```python
from build123d import *

# Parameters (mm, degrees)
F3_R = 0.5
F4_R = 1.25


with BuildPart() as f2:
    # F2: sweep along a path in F1
    with BuildLine(Plane.XY) as f2_path:
        Line((0, 0), (0, 2))
    # F0 (on Front) → F2 (sweep)
    with BuildSketch(Plane.XZ):
        Polygon((-0.5872089498, 2.8263968197), (-2.741335922, 0.904660542), (-2.1541269722, -1.9217362777), (0.5872089498, -2.8263968197), (2.741335922, -0.904660542), (2.1541269722, 1.9217362777), align=None)
    sweep(path=f2_path.line)

    # F3
    f3_edges = [f2.edges().sort_by_distance(p)[0] for p in [
        (-2.447731, 0, -0.508538),
        (-1.664272, 0, 1.865529),
        (0.783459, 0, 2.374067),
        (2.447731, 0, 0.508538),
        (1.664272, 0, -1.865529),
        (-0.783459, 0, -2.374067),
        (-1.664272, 2, 1.865529),
        (0.783459, 2, 2.374067),
        (2.447731, 2, 0.508538),
        (1.664272, 2, -1.865529),
        (-0.783459, 2, -2.374067),
        (-2.447731, 2, -0.508538),
    ]]
    fillet(f3_edges, radius=F3_R)

    # F6: sweep along a path in F5
    with BuildLine(Plane.XY) as f6_path:
        Line((0, -0.6415657117), (0, 2.5134647731))
    # F4 (on Front) → F6 (sweep, cut)
    with BuildSketch(Plane.XZ):
        Circle(F4_R)
    sweep(path=f6_path.line, mode=Mode.SUBTRACT)


solid = f2.part
```
Geometry: final body of the model. Coordinates: model frame, mm. Round coordinates to 2 decimals unless told otherwise and drop trailing zeros. Loops run counter-clockwise (first coordinate to the right, second up) from the corner with the lowest first, then second, coordinate; pieces in that order, holes last. Notation, with made-up numbers: (18.25, 78) -> (66.25, 78) arc R8 cw to (66.25, 85) -> close; hole circle Ø3 at (53, -26). An arc over 180 degrees is marked (long way). Use one line per item in the form item = value. Start each with the question number.
1) Draft query along X for faces 1 (the cylindrical face through (0.72, 0.15, 2.245)), 2 (the cylindrical face through (-0.27, 1.01, 1.22)), 3 (the cylindrical face through (-2.304, 1.85, -0.499)). Return one class per face: released by +X, released by -X, zero draft, split by the parting line, or undercut.
2) Section B-B on y = 0.4. Output: boundary loops of the cut face in (x, z), then the cut area to 3 significant figures.
3) Line query: L1, parallel to Z at x = 0.4, y = 0.45; L2, parallel to Z at x = 0, y = 1; L3, parallel to X at y = 0.65, z = -0.2. Output: solid intervals per line, ascending.
4) Section A-A on y = 0.75. Output: boundary loops of the cut face in (x, z).
5) First-contact query: P1, Ø1, axis at x = 2, y = 2, coming from the -Z side. Flat tip, straight axial feed; report the tip coordinate or a pass-through.
Response:
q1.face_1 = released by +X
q1.face_2 = undercut
q1.face_3 = released by -X
q2.outline = (-2.73, 0.9) -> (-2.15, -1.91) -> (0.58, -2.81) -> (2.73, -0.9) -> (2.15, 1.91) -> (-0.58, 2.81) -> close; hole circle Ø2.5 at (0, 0)
q2.area = 16.6 mm^2
q3.L1 = -2.76 to -1.18, 1.18 to 2.5
q3.L2 = -2.63 to -1.25, 1.25 to 2.63
q3.L3 = -2.51 to -1.23, 1.23 to 2.59
q4.outline = (-2.74, 0.9) -> (-2.15, -1.92) -> (0.59, -2.83) -> (2.74, -0.9) -> (2.15, 1.92) -> (-0.59, 2.83) -> close; hole circle Ø2.5 at (0, 0)
q5.P1 = -1.87
